The listing builds one solid part. Answer for the finished solid, in the listing's coordinates (mm). Face numbers are marked on the shaded views. Round coordinates to 2 decimals unless told otherwise and drop trailing zeros. Order: outer loops, then holes, each group sorted by start corner. A loop starts at its lowest first (then second) coordinate and runs counter-clockwise, first axis right, second up. Notation, with made-up numbers: (-17, 85) -> (5, 85) arc R23 ccw to (5, 97) -> close; hole circle Ø6 at (16.5, -16.5). An arc over 180 degrees is marked (long way). Answer in a Markdown table with one row per item. Add a question column.
```python
from build123d import *

# Parameters (mm, degrees)
SKETCH1_W           = 28.47
SKETCH1_H           = 29.97
BOSS_EXTRUDE1_DEPTH = 5
CUT_EXTRUDE1_REACH  = 7
SKETCH2_R           = 4.5
SKETCH4_W           = 28.47
SKETCH4_H           = 29.97
SKETCH4_W_2         = 26.07
SKETCH4_H_2         = 27.57
BOSS_EXTRUDE2_DEPTH = 2
SKETCH7_R           = 6.25
CUT_EXTRUDE5_DEPTH  = 1
FILLET1_R           = 3
SKETCH8_W           = 5
SKETCH8_H           = 1.6
CUT_EXTRUDE6_DEPTH  = 1.2


with BuildPart() as part:
    # Sketch1 → Boss-Extrude1 (new body)
    with BuildSketch(Plane(origin=(0, 0, 0), x_dir=(1, 0, 0), z_dir=(0, 1, 0))):
        Rectangle(SKETCH1_W, SKETCH1_H)
    extrude(amount=-BOSS_EXTRUDE1_DEPTH)

    # Sketch2 → Cut-Extrude1 (cut, up to next)
    with BuildSketch(Plane(origin=(0, 0, 0), x_dir=(1, 0, 0), z_dir=(0, 1, 0)), mode=Mode.PRIVATE) as cut_extrude1_sk1:
        Circle(SKETCH2_R)
    cut_extrude1_tool1 = extrude(cut_extrude1_sk1.sketch, amount=-CUT_EXTRUDE1_REACH, mode=Mode.PRIVATE) & part.part
    add(cut_extrude1_tool1.solids().sort_by_distance((0, 0, 0))[0], mode=Mode.SUBTRACT)

    # Sketch4 → Boss-Extrude2 (add)
    with BuildSketch(Plane(origin=(0, 0, 0), x_dir=(1, 0, 0), z_dir=(0, 1, 0))):
        Rectangle(SKETCH4_W, SKETCH4_H)
        Rectangle(SKETCH4_W_2, SKETCH4_H_2, mode=Mode.SUBTRACT)
    extrude(amount=BOSS_EXTRUDE2_DEPTH)

    # Sketch7 → Cut-Extrude5 (cut)
    with BuildSketch(Plane(origin=(0, 0, 0), x_dir=(1, 0, 0), z_dir=(0, 1, 0))):
        Circle(SKETCH7_R)
    extrude(amount=-CUT_EXTRUDE5_DEPTH, mode=Mode.SUBTRACT)

    # Fillet1
    fillet1_edges = [part.edges().sort_by_distance(p)[0] for p in [
        (13.035, 1, -13.785),
        (-13.035, 1, -13.785),
        (-13.035, 1, 13.785),
        (13.035, 1, 13.785),
    ]]
    fillet(fillet1_edges, radius=FILLET1_R)

    # Sketch8 → Cut-Extrude6 (cut)
    with BuildSketch(Plane(origin=(0, 0, -14.985), x_dir=(-1, 0, 0), z_dir=(0, 0, -1))):
        with Locations((0, 1.2)):
            Rectangle(SKETCH8_W, SKETCH8_H)
    extrude(amount=-CUT_EXTRUDE6_DEPTH, mode=Mode.SUBTRACT)


solid = part.part
```
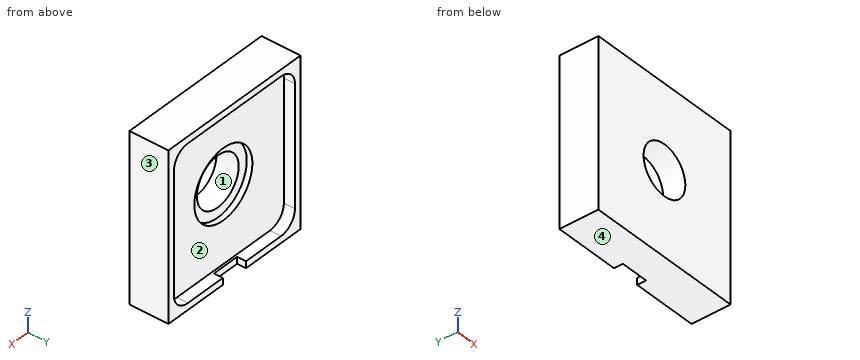
1. The part is cut by section D-D (z = 5). Give the vertices of the cut face in (x, y) (3 decimals), then the cut area to 3 significant figures.
2. The mould has two halves that part along Z. Classify the marked faces 1, 2, 3 and 4: released by +Z, released by -Z, zero draft, split by the parting line, or undercut.
3. The part is cut by section C-C (y = -4). Give the vertices of the cut face in (x, z) (3 decimals), then the cut area to 3 significant figures.
4. The part is cut by section A-A (x = 0). Give the vertices of the cut face in (y, z) (3 decimals).
5. The part is cut by section B-B (z = 0). Give the vertices of the cut face in (x, y) (3 decimals).
6. Straight lines are drawn through the part: line 1 along Z through (x, y) = (-6.5, 1) (3 decimals); line 2 along X through (y, z) = (-0.3, 0) (3 decimals); line 3 along Z through (x, y) = (0, -3.3) (3 decimals). For each, find the intervals that lie inside material, in ascending order.
7. Each of these flat-tipped pins is pushed along its axis until it touches: pin 1 (6 mm diameter, centred on x = 3, z = -1, fed in from +Y); pin 2 (1.3 mm diameter, centred on x = 1, z = -14.5, fed in from +Y); pin 3 (6 mm diameter, centred on x = 8, z = -5.5, fed in from +Y). Where does it stop, or does it pass through?
Report:
| question | item | result |
|---|---|---|
| 1 | outline | (-14.235, -5) -> (14.235, -5) -> (14.235, 2) -> (13.035, 2) -> (13.035, 0) -> (3.75, 0) -> (3.75, -1) -> (-3.75, -1) -> (-3.75, 0) -> (-13.035, 0) -> (-13.035, 2) -> (-14.235, 2) -> close |
| 1 | area | 140 mm^2 |
| 2 | face 1 | undercut |
| 2 | face 2 | undercut |
| 2 | face 3 | zero draft |
| 2 | face 4 | released by -Z |
| 3 | outline | (-14.235, -14.985) -> (14.235, -14.985) -> (14.235, 14.985) -> (-14.235, 14.985) -> close; hole circle Ø9 at (0, 0) |
| 3 | area | 790 mm^2 |
| 4 | outline | (-5, -14.985) -> (0.4, -14.985) -> (0.4, -13.785) -> (0, -13.785) -> (0, -6.25) -> (-1, -6.25) -> (-1, -4.5) -> (-5, -4.5) -> close; (-5, 4.5) -> (-1, 4.5) -> (-1, 6.25) -> (0, 6.25) -> (0, 13.785) -> (2, 13.785) -> (2, 14.985) -> (-5, 14.985) -> close |
| 5 | outline | (-14.235, -5) -> (-4.5, -5) -> (-4.5, -1) -> (-6.25, -1) -> (-6.25, 0) -> (-13.035, 0) -> (-13.035, 2) -> (-14.235, 2) -> close; (4.5, -5) -> (14.235, -5) -> (14.235, 2) -> (13.035, 2) -> (13.035, 0) -> (6.25, 0) -> (6.25, -1) -> (4.5, -1) -> close |
| 6 | line 1 | z = -14.985 to -13.785, 13.785 to 14.985 |
| 6 | line 2 | x = -14.235 to -6.25, 6.25 to 14.235 |
| 6 | line 3 | z = -14.985 to -4.5, 4.5 to 14.985 |
| 7 | pin 1 | stops at y = -1 |
| 7 | pin 2 | stops at y = 0.4 |
| 7 | pin 3 | stops at y = 0 |
